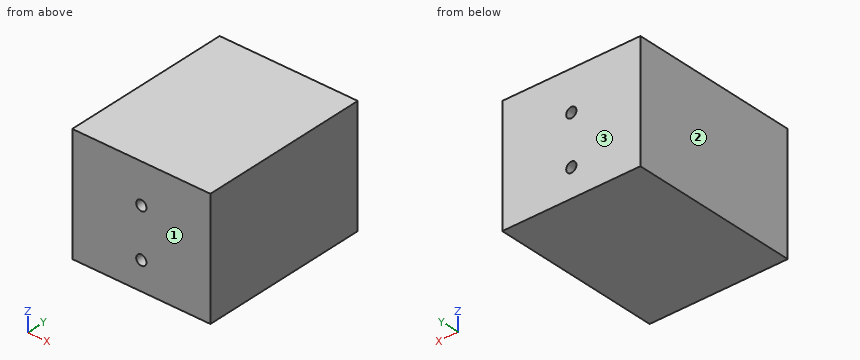
```python
from build123d import *

# Parameters (mm, degrees)
SKETCH1_W           = 47.27
SKETCH1_H           = 58.4
BOSS_EXTRUDE1_DEPTH = 40.2
SKETCH4_R           = 1.75
CUT_EXTRUDE2_DEPTH  = 60


with BuildPart() as part:
    # Sketch1 → Boss-Extrude1 (new body)
    with BuildSketch(Plane.XY):
        with Locations((-23.691836225, -14.070929403)):
            Rectangle(SKETCH1_W, SKETCH1_H)
    extrude(amount=BOSS_EXTRUDE1_DEPTH)

    # Sketch4 → Cut-Extrude2 (cut)
    with BuildSketch(Plane.XZ.offset(43.270929403)):
        with Locations(Location((-23.691836225, 9.702218518, 0), (0, 0, 270))):
            Circle(SKETCH4_R)
        with Locations(Location((-23.691836225, 26.573715394, 0), (0, 0, 270))):
            Circle(SKETCH4_R)
    extrude(amount=-CUT_EXTRUDE2_DEPTH, mode=Mode.SUBTRACT)


solid = part.part
```
CAD build for the part. Positions are in the model's coordinates, mm. Face numbers are marked on the shaded views. Coordinates: 2 decimals unless noted, no trailing zeros. Use a Markdown table: item, result. Add a question column.
(1) Flat gauge pin, fed straight in: pin 1 (3 mm diameter, centred on x = -23.69, z = 26.57, fed in from +Y). Where does the tip first touch, or does it go through?
(2) Drill centre lines: line 1 along Z through (x, y) = (-24.5, 6); line 2 along X through (y, z) = (4.5, 10.5); line 3 along X through (y, z) = (-23.5, 25.5). Where is each one in solid material? Low to high. Write a range as [from, to].
(3) Pull direction Y, two halves, no side cores. Call the marked faces 1, 2 and 3: +Y half, -Y half, draft (parallel to the pull), parting line (faces both ways), or undercut.
Solved:
| question | item | result |
|---|---|---|
| 1 | pin 1 | passes through |
| 2 | line 1 | z = [0, 8.15], [11.25, 25.02], [28.13, 40.2] |
| 2 | line 2 | x = [-47.33, -25.25], [-22.13, -0.06] |
| 2 | line 3 | x = [-47.33, -25.07], [-22.31, -0.06] |
| 3 | face 1 | -Y half |
| 3 | face 2 | draft |
| 3 | face 3 | +Y half |
